Part model, mm, in its own coordinate system. Face numbers are marked on the shaded views. A direction names the side the tool comes from. Coordinates: 2 decimals unless noted, no trailing zeros. Loops run counter-clockwise (first coordinate to the right, second up) from the corner with the lowest first, then second, coordinate; pieces in that order, holes last. Notation, with made-up numbers: M 63,4.25 L 88,4.25 A12 ccw 88,9.25 Z; hole C 2,-35.5 d8. An arc over 180 degrees is marked long. Use a Markdown table: item, result. Add a question column.
1) Tool access for the marked faces 1 and 2: list every direction of +Z, -Z, +X, -X, +Y, -Y with a clear straight run to the whole face (end or side of a thin tool).
2) Band-saw the part on A-A (x = 143.5). List the corners of the cut face in (y, z) (3 decimals).
3) Band-saw the part on B-B (y = 258.5). List the corners of the cut face in (x, z) (3 decimals), plus the area to 3 significant figures.
4) Band-saw the part on C-C (x = 240). List the corners of the cut face in (y, z) (3 decimals), plus the area to 3 significant figures.
5) Wall check: probe 1 along Z at (x, y) = (127, 275.35); probe 2 along Y at (x, z) = (292.1, -0.8); probe 3 along Y at (x, z) = (234, -7) (3 decimals). Give the ranges that are in metal, low to high. Write a range as from..to.
6) Pin check, flat tips, straight feed: pin 1 Ø10 at (y, z) = (70, -9.5) entering from -X; pin 2 Ø1.5 at (x, z) = (79, -18.5) entering from -Y; pin 3 Ø12 at (x, y) = (73.5, 229.5) entering from -Z (3 decimals). Stop position of each tip, or through.
Autodesk Inventor part; units mm, degrees
ref_plane "YZ Plane" through (0, 0, 0) normal (1, 0, 0) x (0, 1, 0)
ref_plane "XZ Plane" through (0, 0, 0) normal (0, 1, 0) x (-1, 0, 0)
ref_plane "XY Plane" through (0, 0, 0) normal (0, 0, 1) x (1, 0, 0)
sketch "Sketch1" plane through (0, 0, 0) normal (1, 0, 0) x (0, 1, 0)
  line L0 (0, 0) -> (276.225, 0)
  line L1 (276.225, 0) -> (276.225, -25.4)
  dimension "d0" = 25.4
  dimension "d1" = 276.225
contour flange "Contour Flange1" sketch "Sketch1" thickness 3.175 bend radius 3.175 width 304.8 along (1, 0, 0) mid plane no both sides no wall seen from (0, 138.1125, 0) lies toward (0, 0, -1) curves L0 L1
bend "Bend1"
corner "Corner1"
sketch "Sketch2" plane through (0, 0, 0) normal (0, 0, 1) x (1, 0, 0)
  line L0 (304.8, 0) -> (304.8, 269.875)
  line L1 (304.8, 0) -> (0, 53.7445)
  line L2 (0, 0) -> (0, 269.875)
  line L3 (0, 269.875) -> (304.8, 269.875)
  line L4 (0, 0) -> (0, 269.875)
  line L5 (304.8, 0) -> (0, 0)
  line L6 (304.8, 269.875) -> (304.8, 0)
  dimension "d13" = 10
extrude "Cut1" cut sketch "Sketch2" against normal blind 3.175 contours L5 L2 L1
sketch "Sketch3" plane through (0, 276.225, -25.4) normal (0, 1, 0) x (1, 0, 0)
  line L0 (304.8, -22.225) -> (282.575, 0)
  line L1 (0, 0) -> (304.8, 0)
  line L2 (304.8, 0) -> (304.8, -19.05)
  line L3 (304.8, 0) -> (304.8, -22.225)
  point P0 (0, -25.4)
  dimension "d16" = 45
extrude "Cut2" cut sketch "Sketch3" against normal through all
sketch "Sketch4" plane through (0, 269.875, 0) normal (0, 0, 1) x (1, 0, 0)
  line L0 (304.8, 0) -> (304.8, -269.875)
  point P0 (0, -269.875)
  point P1 (292.1, -196.85)
  point P2 (292.1, -146.05)
  point P3 (292.1, -95.25)
  point P4 (292.1, -44.45)
  dimension "d19" = 73.025
  dimension "d20" = 12.7
  dimension "d23" = 50.8
hole "Hole1" at (292.1, 73.025, 0) at (292.1, 123.825, 0) at (292.1, 174.625, 0) at (292.1, 225.425, 0) direction (0, 0, -1) diameter 5.105 end through all
sketch "Sketch5" plane through (0, 276.225, -6.35) normal (0, 1, 0) x (1, 0, 0)
  line L0 (0, 19.05) -> (282.575, 19.05)
  line L1 (0, 0) -> (0, 19.05)
  point P0 (0, -6.35)
  point P1 (25.4, 9.525)
  point P2 (76.2, 9.525)
  point P3 (127, 9.525)
  point P4 (177.8, 9.525)
  point P5 (228.6, 9.525)
  point P6 (279.4, 9.525)
  dimension "d35" = 9.525
  dimension "d36" = 25.4
  dimension "d39" = 50.8
hole "Hole2" at (25.4, 276.225, -15.875) at (76.2, 276.225, -15.875) at (127, 276.225, -15.875) at (177.8, 276.225, -15.875) at (228.6, 276.225, -15.875) at (279.4, 276.225, -15.875) direction (0, -1, 0) diameter 5.105 end through all
sketch "Sketch6" plane through (0, 269.875, 0) normal (0, 0, 1) x (1, 0, 0)
  circle A0 centre (52.3434, -199.5683) radius 4.7625
  line L0 (0, -216.1305) -> (304.8, -269.875)
  line L1 (0, -216.1305) -> (0, 0)
  point P0 (0, -269.875)
  dimension "d51" = 9.525
  dimension "d52" = 25.4
  dimension "d53" = 52.3434
extrude "Cut3" cut sketch "Sketch6" against normal blind 3.175
equation "\"d14\" = Thickness"
equation "\"d17\" = Thickness"
equation "\"d33\" = Thickness"
equation "\"d54\" = Thickness"
equation "\"d2\" = Thickness"
equation "\"d3\" = BendReliefWidth"
equation "\"d4\" = BendReliefDepth"
equation "\"d5\" = MinimumRemnant"
equation "\"d6\" = TransitionRadius"
equation "\"d8\" = BendRadius"
equation "\"d10\" = CornerReliefSize"
equation "\"d11\" = GapSize"
equation "\"d12\" = JacobiRadiusSize"
equation "\"BendRadius\" = Thickness"
equation "\"BendReliefWidth\" = Thickness"
equation "\"BendReliefDepth\" = 0.5 * Thickness"
equation "\"CornerReliefSize\" = 4 * Thickness"
equation "\"MinimumRemnant\" = 2 * Thickness"
equation "\"TransitionRadius\" = BendRadius"
equation "\"JacobiRadiusSize\" = BendRadius"
equation "\"GapSize\" = Thickness"
properties part number "SIDE_INTAKE_LEXAN" material "Polycarbonate, PC 1000, Clear"
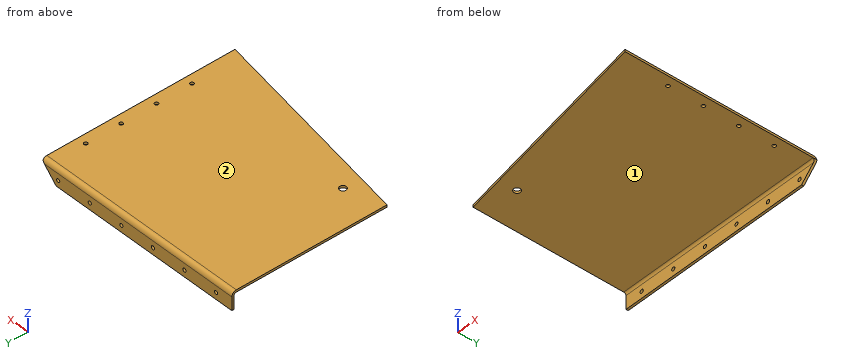
Entries:
| question | item | result |
|---|---|---|
| 1 | face 1 | -Z, +X, -X, -Y |
| 1 | face 2 | +Z, +X, -X, +Y, -Y |
| 2 | outline | M 28.442,-3.175 L 269.875,-3.175 A3.175 cw 273.05,-6.35 L 273.05,-25.4 L 276.225,-25.4 L 276.225,-6.35 A6.35 ccw 269.875,0 L 28.442,0 Z |
| 3 | outline | M 0,-3.175 L 304.8,-3.175 L 304.8,0 L 0,0 Z |
| 3 | area | 968 mm2 |
| 4 | outline | M 11.426,-3.175 L 269.875,-3.175 A3.175 cw 273.05,-6.35 L 273.05,-25.4 L 276.225,-25.4 L 276.225,-6.35 A6.35 ccw 269.875,0 L 11.426,0 Z |
| 4 | area | 905 mm2 |
| 5 | probe 1 | -25.4..-18.43, -13.32..-3.13 |
| 5 | probe 2 | 2.24..70.47, 75.58..121.27, 126.38..172.07, 177.18..222.87, 227.98..272.96 |
| 5 | probe 3 | 273.05..276.225 |
| 6 | pin 1 | through |
| 6 | pin 2 | y = 273.05 |
| 6 | pin 3 | z = -3.175 |
